```python
from build123d import *

# Parameters (mm, degrees)
SKETCH5_W                    = 475.54896
SKETCH5_H                    = 260.35
BASE_FLANGE1_DEPTH           = 3.175
EDGE_FLANGE1_DEPTH           = 366.48136
EDGE_FLANGE2_STRIP_W         = 19.05
EDGE_FLANGE2_STRIP_H         = 3.175
EDGE_FLANGE2_STRIP_CUT_DEPTH = 260.35
EDGE_FLANGE2_DEPTH           = 260.35
EDGE_FLANGE3_DEPTH           = 260.35
CUT_EXTRUDE1_DEPTH           = 279.698003441
CUT_EXTRUDE1_DEPTH_BACK      = 279.698003441
SKETCH16_W                   = 336.938395151
SKETCH16_H                   = 122.280894257


# Sheet-metal steps are written as plain solids
with BuildPart() as part:
    # Sketch5 → Base-Flange1 (new body)
    with BuildSketch(Plane(origin=(0, 0, 0), x_dir=(1, 0, 0), z_dir=(0, 1, 0))):
        Rectangle(SKETCH5_W, SKETCH5_H)
    extrude(amount=-BASE_FLANGE1_DEPTH)

    # Edge-Flange1 section (across the edge) → Edge-Flange1 (add)
    with BuildSketch(Plane(origin=(-237.77448, 0, 133.35), x_dir=(0, 0, -1), z_dir=(1, 0, 0))):
        with BuildLine():
            Line((-3.175, 3.175), (-3.175, 15.875))
            Line((-3.175, 15.875), (0, 15.875))
            Line((0, 15.875), (0, 3.175))
            ThreePointArc((0, 3.175), (0.92993597, 0.92993597), (3.175, 0))
            Line((3.175, 0), (3.175, -3.175))
            ThreePointArc((3.175, -3.175), (-1.315128061, -1.315128061), (-3.175, 3.175))
        make_face()
    extrude(amount=EDGE_FLANGE1_DEPTH)

    # Edge-Flange2 strip (across the edge) → Edge-Flange2 strip cut (cut)
    with BuildSketch(Plane(origin=(237.77448, 0, 130.175), x_dir=(-1, 0, 0), z_dir=(0, 0, -1))):
        with Locations((-3.175, -1.5875)):
            Rectangle(EDGE_FLANGE2_STRIP_W, EDGE_FLANGE2_STRIP_H)
    extrude(amount=EDGE_FLANGE2_STRIP_CUT_DEPTH, mode=Mode.SUBTRACT)

    # Edge-Flange2 section (across the edge) → Edge-Flange2 (add)
    with BuildSketch(Plane(origin=(237.77448, 0, 130.175), x_dir=(-1, 0, 0), z_dir=(0, 0, -1))):
        with BuildLine():
            Line((0, 3.175), (0, 22.225))
            Line((0, 22.225), (3.175, 22.225))
            Line((3.175, 22.225), (3.175, 3.175))
            ThreePointArc((3.175, 3.175), (4.10493597, 0.92993597), (6.35, 0))
            Line((6.35, 0), (6.35, -3.175))
            ThreePointArc((6.35, -3.175), (1.859871939, -1.315128061), (0, 3.175))
        make_face()
    extrude(amount=EDGE_FLANGE2_DEPTH)

    # Edge-Flange3 section (across the edge) → Edge-Flange3 (add)
    with BuildSketch(Plane(origin=(-238.77448, 0, -130.175), x_dir=(1, 0, 0), z_dir=(0, 0, 1))):
        with BuildLine():
            Line((-3.175, 1), (-3.175, 22.225))
            Line((-3.175, 22.225), (0, 22.225))
            Line((0, 22.225), (0, 1))
            ThreePointArc((0, 1), (0.292893219, 0.292893219), (1, 0))
            Line((1, 0), (1, -3.175))
            ThreePointArc((1, -3.175), (-1.952170811, -1.952170811), (-3.175, 1))
        make_face()
    extrude(amount=EDGE_FLANGE3_DEPTH)

    # Sketch16 → Cut-Extrude1 (cut, two sides: drawn at the far end of the back side and taken through both)
    with BuildSketch(Plane(origin=(0, 0, 0), x_dir=(1, 0, 0), z_dir=(0, 1, 0)).offset(-CUT_EXTRUDE1_DEPTH_BACK)):
        with Locations((168.469197576, 127.815447129)):
            Rectangle(SKETCH16_W, SKETCH16_H)
    extrude(amount=CUT_EXTRUDE1_DEPTH + CUT_EXTRUDE1_DEPTH_BACK, mode=Mode.SUBTRACT)


solid = part.part
```
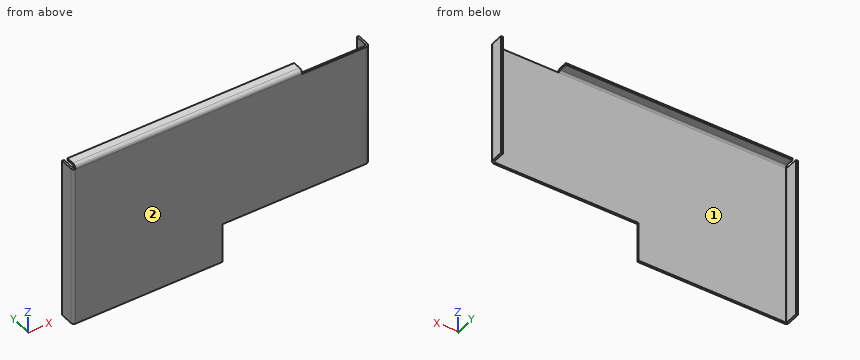
Can you work these out from the model? Positions are in its coordinate system, mm. Face numbers are marked on the shaded views. Round coordinates to 2 decimals unless told otherwise and drop trailing zeros. Loops run counter-clockwise (first coordinate to the right, second up) from the corner with the lowest first, then second, coordinate; pieces in that order, holes last.
Item 1: If we mould it in two halves opening along X, with no side actions, what happens to the marked faces 1 and 2? For each: +X half, -X half, draft (parallel to the pull), parting line (faces both ways), or undercut.
Item 2: Will these pins go through, and if not, where does the flat tip stop? pin 1 Ø5 at (y, z) = (10, 134) entering from -X; pin 2 Ø6 at (y, z) = (3.5, -101.5) entering from +X; pin 3 Ø8 at (x, y) = (-13.5, 13) entering from -Z.
Item 3: Suppose I cut it at B-B, the plane x = -197. Write out the boundary of the cut face in (y, z) (3 decimals).
Item 4: Suppose I cut it at A-A, the plane y = 7. Write out the boundary of the cut face in (x, z) (3 decimals).
Item 5: Please list where these lines run through material, in increasing order: L1, parallel to X at y = 12.5, z = 79; L2, parallel to Y at x = 81.5, z = 77 (3 decimals); L3, parallel to X at y = 15.75, z = -70.
Item 6: Suppose I cut it at C-C, the plane z = -103. Write out the boundary of the cut face in (x, y) (3 decimals).
Item 7: Suppose I cut it at D-D, the plane z = 48. Write out the boundary of the cut face in (x, y) (3 decimals), then the cut area to 3 significant figures.
Reported:
1. face 1: undercut
1. face 2: draft
2. pin 1: stops at x = -237.77
2. pin 2: stops at x = -238.64
2. pin 3: stops at z = 133.35
3. outline: (-3.175, -130.175) - (0, -130.175) - (0, 130.175) arc R3.175 cw to (3.175, 133.35) - (15.875, 133.35) - (15.875, 136.525) - (3.175, 136.525) arc R6.35 ccw to (-3.175, 130.175) - close
4. outline: (-241.949, -130.175) - (-238.774, -130.175) - (-238.774, 130.175) - (-241.949, 130.175) - close; (-237.774, 133.35) - (128.707, 133.35) - (128.707, 136.525) - (-237.774, 136.525) - close; (234.599, -66.675) - (237.774, -66.675) - (237.774, 130.175) - (234.599, 130.175) - close
5. L1: x = -241.95 to -238.77, 234.6 to 237.77
5. L2: y = -3.175 to 0
5. L3: x = -241.95 to -238.77
6. outline: (-241.949, 1) arc R4.175 ccw to (-237.774, -3.175) - (0, -3.175) - (0, 0) - (-237.774, 0) arc R1 cw to (-238.774, 1) - (-238.774, 22.225) - (-241.949, 22.225) - close
7. outline: (-241.949, 1) arc R4.175 ccw to (-237.774, -3.175) - (231.424, -3.175) arc R6.35 ccw to (237.774, 3.175) - (237.774, 22.225) - (234.599, 22.225) - (234.599, 3.175) arc R3.175 cw to (231.424, 0) - (-237.774, 0) arc R1 cw to (-238.774, 1) - (-238.774, 22.225) - (-241.949, 22.225) - close
7. area: 1,650 mm2
